from build123d import *
from build123d.topology import SkipClean

# Parameters (mm, degrees)
SKETCH_1_R          = 6
SKETCH_1_R_2        = 5.15
EXTRUDE_3_DEPTH     = 4
SKETCH_2_R          = 6
SKETCH_2_R_2        = 5.15
EXTRUDE_4_DEPTH     = 3.5
CUT_EXTRUDE_1_DEPTH = 2
EXTRUDE_5_DEPTH     = 1.6


with BuildPart() as part:
    # 草图1 → 凸台-拉伸3 (new body)
    # profile 1 of 2: a face of its own
    with BuildSketch(Plane(origin=(0, 0, 0), x_dir=(1, 0, 0), z_dir=(0, 1, 0))):
        with BuildLine():
            Line((130, 6), (0, 6))
            ThreePointArc((0, 6), (4.242640687, 4.242640687), (6, 0))
            ThreePointArc((6, 0), (4.242640687, -4.242640687), (0, -6))
            Line((0, -6), (130, -6))
            Line((130, -6), (130, 6))
        make_face()
    # profile 2 of 2: a face of its own
    with BuildSketch(Plane(origin=(0, 0, 0), x_dir=(1, 0, 0), z_dir=(0, 1, 0))):
        Circle(SKETCH_1_R)
        with Locations(Location((0, 0, 0), (0, 0, 270))):
            Circle(SKETCH_1_R_2, mode=Mode.SUBTRACT)
    extrude(amount=EXTRUDE_3_DEPTH)

    # 草图2 → 凸台-拉伸4 (add)
    with BuildSketch(Plane(origin=(0, 4, 0), x_dir=(1, 0, 0), z_dir=(0, 1, 0))):
        with Locations(Location((0, 0, 0), (0, 0, 270))):
            Circle(SKETCH_2_R)
        with Locations(Location((0, 0, 0), (0, 0, 270))):
            Circle(SKETCH_2_R_2, mode=Mode.SUBTRACT)
    extrude(amount=EXTRUDE_4_DEPTH)

    # 草图3 → 切除-拉伸1 (cut)
    with BuildSketch(Plane.XZ):
        Polygon((-2.5, -8.5), (2.5, -8.5), (2.5, -2.5), (6, -2.5), (6, 2.5), (2.5, 2.5), (2.5, 8.5), (-2.5, 8.5), (-2.5, 2.5), (-6, 2.5), (-6, -2.5), (-2.5, -2.5), align=None)
    extrude(amount=-CUT_EXTRUDE_1_DEPTH, mode=Mode.SUBTRACT)

    # 草图4 → 凸台-拉伸5 (add)
    with SkipClean():  # the faces are left unmerged after this step: merging them gives an invalid solid
        with BuildSketch(Plane(origin=(0, 7.5, 0), x_dir=(1, 0, 0), z_dir=(0, 1, 0))):
            with BuildLine():
                ThreePointArc((-4.502499306, -2.5), (-5.15, 0), (-4.502499306, 2.5))
                Line((-4.502499306, 2.5), (-5.454356057, 2.5))
                ThreePointArc((-5.454356057, 2.5), (-6, 0), (-5.454356057, -2.5))
                Line((-5.454356057, -2.5), (-4.502499306, -2.5))
            make_face()
            with BuildLine():
                ThreePointArc((-2.5, 4.502499306), (0, 5.15), (2.5, 4.502499306))
                Line((2.5, 4.502499306), (2.5, 5.454356057))
                ThreePointArc((2.5, 5.454356057), (0, 6), (-2.5, 5.454356057))
                Line((-2.5, 5.454356057), (-2.5, 4.502499306))
            make_face()
            with BuildLine():
                Line((5.440505491, 2.53), (4.485710646, 2.53))
                ThreePointArc((4.485710646, 2.53), (4.981159997, 1.307878085), (5.15, 0))
                ThreePointArc((5.15, 0), (4.985497539, -1.291245247), (4.502499306, -2.5))
                Line((4.502499306, -2.5), (5.454356057, -2.5))
                ThreePointArc((5.454356057, -2.5), (5.862002062, -1.279426367), (6, 0))
                ThreePointArc((6, 0), (5.858456834, 1.295563015), (5.440505491, 2.53))
            make_face()
            with BuildLine():
                Line((2.5, -5.454356057), (2.5, -4.502499306))
                ThreePointArc((2.5, -4.502499306), (0, -5.15), (-2.5, -4.502499306))
                Line((-2.5, -4.502499306), (-2.5, -5.454356057))
                ThreePointArc((-2.5, -5.454356057), (0, -6), (2.5, -5.454356057))
            make_face()
        extrude(amount=EXTRUDE_5_DEPTH)


solid = part.part
Build history of the part. All positions in model axes, mm. A direction names the side the tool comes from. Give positions to 0.01 mm unless a question says otherwise; leave off trailing zeros. Loops run counter-clockwise (first coordinate to the right, second up) from the corner with the lowest first, then second, coordinate; pieces in that order, holes last. Notation, with made-up numbers: (52, 72.25) -> (91, 72.25) arc R21 cw to (91, 111.25) -> close; hole circle Ø4 at (88, 64.25). An arc over 180 degrees is marked (long way). Answer in a Markdown table with one row per item.
Item 1: Flat gauge pins, fed straight in: P1, Ø5, axis at x = 19.5, y = 4.5, coming from the -Z side; P2, Ø1.5, axis at y = 5, z = 3.5, coming from the +X side; P3, Ø0.5, axis at y = 8.5, z = -5, coming from the -X side; P4, Ø1.5, axis at x = -4, z = -3.5, coming from the +Y side. Where does each tip first touch, or does it go through?
Findings below:
| item | result |
|---|---|
| P1 | stops at z = -6 |
| P2 | stops at x = 5.33 |
| P3 | stops at x = -2.5 |
| P4 | stops at y = 7.5 |
Item 2: Slice it at B-B on y = 5.5. Write the cut outline in (x, z).
Findings below:
| item | result |
|---|---|
| outline | circle Ø12 at (0, 0); hole circle Ø10.3 at (0, 0) |
Item 3: Slice it at C-C on x = 84.5. Write the cut outline in (y, z), plus the area to 3 significant figures.
Findings below:
| item | result |
|---|---|
| outline | (0, -6) -> (4, -6) -> (4, 6) -> (0, 6) -> close |
| area | 48.0 mm² |
Item 4: Probe line 1 along Z through (x, y) = (0, 7); line 2 along X through (y, z) = (2.25, -2.5). List the from-to ranges inside material, lowest first. Write a range as [from, to].
Findings below:
| item | result |
|---|---|
| line 1 | z = [-6, -5.15], [5.15, 6] |
| line 2 | x = [-5.45, -4.5], [4.5, 130] |
Item 5: Tool access for faces 1 (the flat face through (4, 7.5, -4)), 2 (the flat face through (-4, 7.5, -4)), 3 (the flat face through (4, 7.5, 4)): list every direction of +Z, -Z, +X, -X, +Y, -Y with a clear straight run to the whole face (end or side of a thin tool).
Findings below:
| item | result |
|---|---|
| face 1 | -Z, +X, +Y |
| face 2 | -Z, -X, +Y |
| face 3 | +Z, +X, +Y |
Item 6: Slice it at A-A on z = 0. Write the cut outline in (x, y), plus the area to 3 significant figures.
Findings below:
| item | result |
|---|---|
| outline | (-6, 2) -> (-5.15, 2) -> (-5.15, 9.1) -> (-6, 9.1) -> close; (5.15, 2) -> (6, 2) -> (6, 0) -> (130, 0) -> (130, 4) -> (6, 4) -> (6, 9.1) -> (5.15, 9.1) -> close |
| area | 508 mm² |
